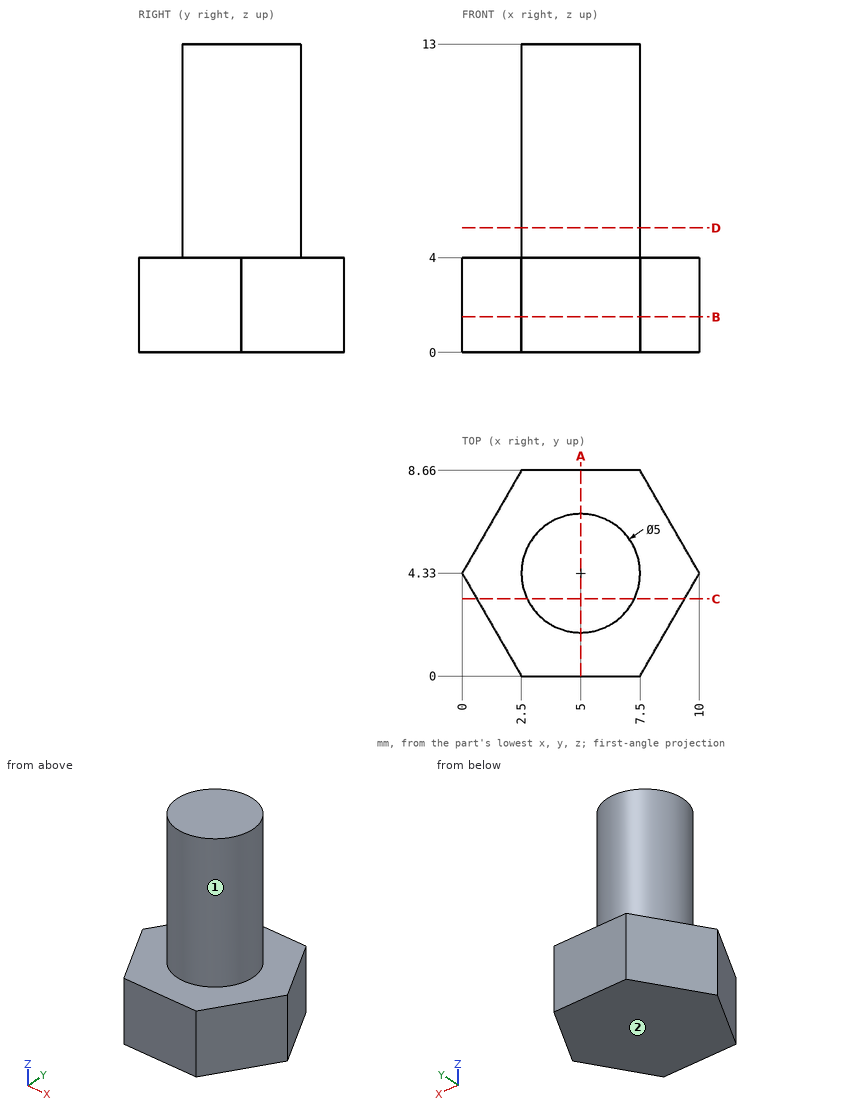
Input: dimensioned drawing with shaded views. Units: mm. Origin: part minimum x, y, z. A direction names the side the tool comes from. Round coordinates to 2 decimals unless told otherwise and drop trailing zeros. Order: outer loops, then holes, each group sorted by start corner. A loop starts at its lowest first (then second) coordinate and runs counter-clockwise, first axis right, second up.
1. Cut plane C-C, the plane y = 3.25. Output: boundary loops of the cut face in (x, z) (1 decimal).
The answers:
outline: (0.6, 0) - (9.4, 0) - (9.4, 4) - (7.3, 4) - (7.3, 13) - (2.7, 13) - (2.7, 4) - (0.6, 4) - close
2. Cut plane A-A, the plane x = 5. Output: boundary loops of the cut face in (y, z).
The answers:
outline: (0, 0) - (8.66, 0) - (8.66, 4) - (6.83, 4) - (6.83, 13) - (1.83, 13) - (1.83, 4) - (0, 4) - close
3. Pin query (flat end, axial travel): P1, Ø4, axis at x = 8, y = 4, coming from the +Z side; P2, Ø1.5, axis at x = 5.5, z = 6.5, coming from the +Y side; P3, Ø5, axis at y = 5.5, z = 7, coming from the +X side; P4, Ø1, axis at x = 5, z = 7, coming from the -Y side. Return the tip coordinate at first contact, or that it passes through.
The answers:
P1: stops at z = 13
P2: stops at y = 6.83
P3: stops at x = 7.5
P4: stops at y = 1.83
4. Cut plane D-D, the plane z = 5.25. Output: boundary loops of the cut face in (x, y), then the cut area to 3 significant figures.
The answers:
outline: circle Ø5 at (5, 4.33)
area: 19.6 mm2
5. Set-up query: the marked faces 1 and 2. Return all of +Z, -Z, +X, -X, +Y, -Y with unobstructed straight access to the full face (end or side cutting, diameter ignored); none if empty.
The answers:
face 1: +Z
face 2: -Z, +X, -X, +Y, -Y
6. Cut plane B-B, the plane z = 1.5. Output: boundary loops of the cut face in (x, y).
The answers:
outline: (0, 4.33) - (2.5, 0) - (7.5, 0) - (10, 4.33) - (7.5, 8.66) - (2.5, 8.66) - close
7. Material intervals for line 1 (Z direction, x = 9, y = 6); line 2 (Y direction, x = 5, z = 8.5); line 3 (X direction, y = 5.5, z = 2.25) (1 decimal), sorted ascending.
The answers:
line 1: z = 0 to 4
line 2: y = 1.83 to 6.83
line 3: x = 0.7 to 9.3
